Could you check a few things on this drawing? It's one solid part, dimensions in mm from its lowest x, y, z. A direction names the side the tool comes from. Give positions to 0.01 mm unless a question says otherwise; leave off trailing zeros. Loops run counter-clockwise (first coordinate to the right, second up) from the corner with the lowest first, then second, coordinate; pieces in that order, holes last. Notation, with made-up numbers: (69.5, 47) -> (112.5, 47) arc R28 ccw to (112.5, 70) -> close; hole circle Ø11 at (88, 74). An arc over 180 degrees is marked (long way). One line per question, with ' | ' between items.
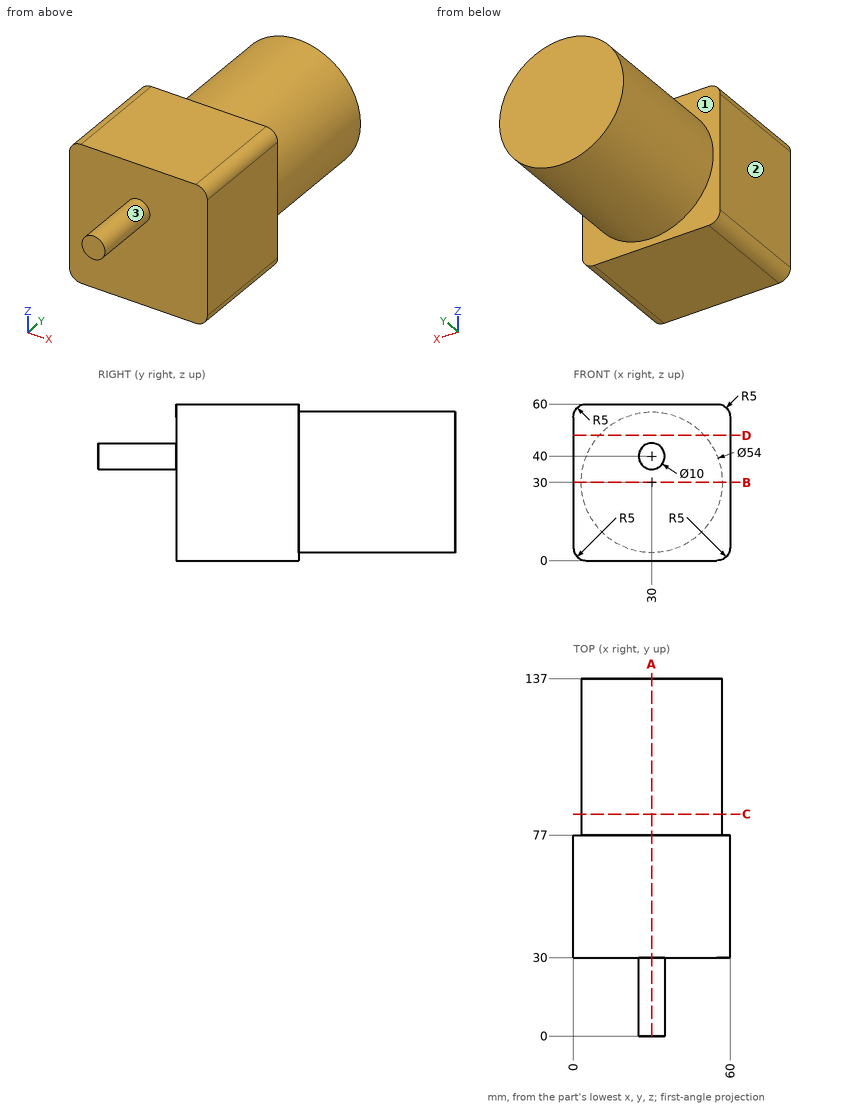
Q1. If we section it at B-B (z = 30): Write out the boundary of the cut face in (x, y).
Entries:
outline: (0, 30) -> (60, 30) -> (60, 77) -> (57, 77) -> (57, 137) -> (3, 137) -> (3, 77) -> (0, 77) -> close
Q2. If we section it at A-A (x = 30): Write out the boundary of the cut face in (y, z), plus the area to 3 significant figures.
Entries:
outline: (0, 35) -> (30, 35) -> (30, 0) -> (77, 0) -> (77, 3) -> (137, 3) -> (137, 57) -> (77, 57) -> (77, 60) -> (30, 60) -> (30, 45) -> (0, 45) -> close | area: 6,360 mm²
Q3. If I drill on probe 1 along Y at (x, z) = (46.5, 9); probe 2 along Y at (x, z) = (7, 12); probe 3 along Z at (x, y) = (24, 115.5), over which ranges is the centre line in solid material (lowest first)? Write a range as from..to.
Entries:
probe 1: 30..137 | probe 2: 30..77 | probe 3: 3.68..56.32
Q4. If we section it at D-D (z = 48): Write out the boundary of the cut face in (x, y).
Entries:
outline: (0, 30) -> (60, 30) -> (60, 77) -> (50.12, 77) -> (50.12, 137) -> (9.88, 137) -> (9.88, 77) -> (0, 77) -> close
Q5. For pin 1 Ø2 at (x, y) = (32.5, 18) entering from +Z; pin 2 Ø4 at (x, y) = (50, 106) entering from -Z; pin 3 Ø10 at (y, z) = (113.5, 48) entering from -X, each with a flat end and sliding along its axis, tell me the tip position at first contact or that it passes through.
Entries:
pin 1: z = 44.77 | pin 2: z = 9.88 | pin 3: x = 6.34
Q6. If we section it at C-C (y = 85): Write out the boundary of the cut face in (x, z), plus the area to 3 significant figures.
Entries:
outline: circle Ø54 at (30, 30) | area: 2,290 mm²
Q7. On a 3-axis mill with a long thin cutter (end or side, diameter ignored), from which of +Z, -Z, +X, -X, +Y, -Y can I reach the whole of each face in a straight line? I mean the marked faces 1, 2 and 3. Say none if no direction works.
Entries:
face 1: +Y | face 2: +Z, -Z, -X, +Y, -Y | face 3: -Y
